CAD build for the part. Positions are in the model's coordinates, mm. A direction names the side the tool comes from. Round coordinates to 2 decimals unless told otherwise and drop trailing zeros. Write each loop counter-clockwise with the first axis right and the second up, starting at its lowest first coordinate (ties: lowest second). Pieces come first, ordered by that corner, then holes. Notation, with made-up numbers: (-23, 29) - (27, 29) arc R11 ccw to (27, 43) - close; hole circle Ø8 at (17.25, 14.25). An arc over 180 degrees is marked (long way). Put each result on its own line as item: value. Start each with the question number.
Item 1: Pin check, flat tips, straight feed: pin 1 Ø12 at (x, y) = (-25.5, 8.5) entering from +Z; pin 2 Ø7 at (y, z) = (-9.5, 67.5) entering from +X; pin 3 Ø6 at (x, z) = (50.5, 28) entering from -Y. Stop position of each tip, or through.
Item 2: Cut at D-D (z = 24). Give the cut face in (x, y), and give its area (3 significant figures).
Item 3: Cut at B-B (z = 10.5). Give the cut face in (x, y).
Item 4: Drill centre lines: line 1 (Z direction, x = 93.5, y = -9); line 2 (Z direction, x = -33.5, y = 40); line 3 (X direction, y = 29, z = 7). Where is each one in solid material? Low to high. Write a range as from..to.
Item 5: Cut at C-C (x = 50). Give the cut face in (y, z).
Item 6: Cut at A-A (y = -20). Give the cut face in (x, z), and give its area (3 significant figures).
Item 7: 3-axis set-ups, long thin cutter, end or side, ignore diameter. For faces 1 (the flat face through (69, 0, 59)), 2 (the flat face through (41.847, -13, 24)), 3 (the flat face through (69, -25.4, 59)), 4 (the flat face through (65.602, -1, 2)): which of +Z, -Z, +X, -X, +Y, -Y reach the whole face in a straight line?
Item 8: Mould opens along X. For faces 5 (the flat face through (-1, -1, -16.733)), 6 (the cylindrical face through (75.418, -12.522, 53.684)), 7 (the flat face through (106.255, -13, 71)) say: released by +X, released by -X, zero draft, split by the parting line, or undercut.
```python
from build123d import *

# Parameters (mm, degrees)
F1_DEPTH = 63.5
F2_DEPTH = 25.4


with BuildPart() as f1:
    # F0 (on Front) → F1 (new body, symmetric)
    with BuildSketch(Plane.XZ):
        Polygon((65.602288, -16.733009), (65.602288, 16.733009), (41.847356, 16.733009), (-65.602288, 16.733009), (-65.602288, -16.733009), align=None)
    extrude(amount=F1_DEPTH, both=True)

    # F0 (on Front) → F2 (join)
    with BuildSketch(Plane.XZ):
        with BuildLine():
            Line((41.847356, 16.733009), (65.602288, 16.733009))
            Line((65.602288, 16.733009), (65.602288, 31.725151))
            ThreePointArc((65.602288, 31.725151), (75.681663, 53.916889), (99.024929, 60.928233))
            Line((99.024929, 60.928233), (106.255405, 59.949448))
            Line((106.255405, 59.949448), (106.255405, 82.992167))
            Line((106.255405, 82.992167), (113.11721, 82.992167))
            Line((113.11721, 82.992167), (102.211555, 84.468458))
            ThreePointArc((102.211555, 84.468458), (60.051584, 71.805361), (41.847356, 31.725151))
            Line((41.847356, 31.725151), (41.847356, 16.733009))
        make_face()
    extrude(amount=F2_DEPTH)


solid = f1.part
```
Output values:
1. pin 1: z = 16.73
1. pin 2: x = 106.26
1. pin 3: y = -25.4
2. outline: (41.85, -25.4) - (65.6, -25.4) - (65.6, 0) - (41.85, 0) - close
2. area: 603 mm2
3. outline: (-65.6, -63.5) - (65.6, -63.5) - (65.6, 63.5) - (-65.6, 63.5) - close
4. line 1: 61.15..84.93
4. line 2: -16.73..16.73
4. line 3: -65.6..65.6
5. outline: (-63.5, -16.73) - (63.5, -16.73) - (63.5, 16.73) - (0, 16.73) - (0, 60.03) - (-25.4, 60.03) - (-25.4, 16.73) - (-63.5, 16.73) - close
6. outline: (-65.6, -16.73) - (65.6, -16.73) - (65.6, 31.73) arc R29.47 cw to (99.02, 60.93) - (106.26, 59.95) - (106.26, 82.99) - (113.12, 82.99) - (102.21, 84.47) arc R53.22 ccw to (41.85, 31.73) - (41.85, 16.73) - (-65.6, 16.73) - close
6. area: 6,560 mm2
7. face 1: +Z, +X, -X, +Y
7. face 2: +Z, -X, +Y, -Y
7. face 3: +Z, +X, -X, -Y
7. face 4: -Z, +X, +Y, -Y
8. face 5: zero draft
8. face 6: undercut
8. face 7: released by +X
